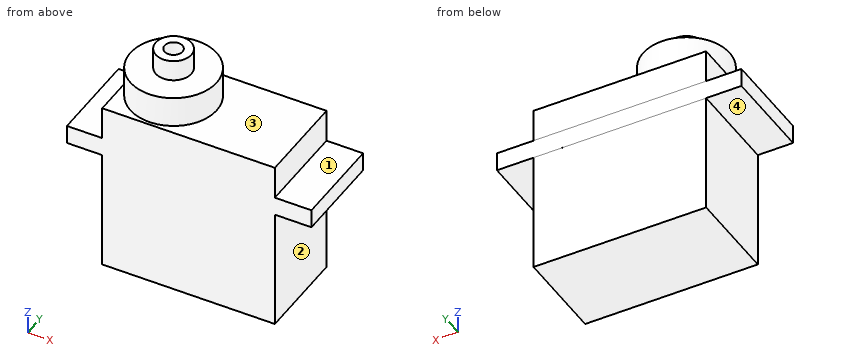
Solid Edge part; units mm, degrees
sketch "Sketch1" plane through (0, 0, 0) normal (0, 0, 1) x (1, 0, 0)
  line L0 (3.8592, 44.8625) -> (26.6354, 44.8625)
  line L1 (26.6354, 44.8625) -> (26.6354, 57.0462)
  line L2 (3.8592, 57.0462) -> (26.6354, 57.0462)
  line L3 (3.8592, 44.8625) -> (3.8592, 57.0462)
extrude "Ajout_matière_1" add sketch "Sketch1" against normal blind 16.002 and the other way blind 6.858
sketch "Sketch2" plane through (26.6354, 50.9544, -4.572) normal (1, 0, 0) x (0, 1, 0)
  line L0 (-5.4864, 7.0592) -> (6.0919, 7.0592)
  line L1 (6.0919, 7.0592) -> (6.0919, 4.572)
  line L2 (6.0919, 4.572) -> (-6.0919, 4.572)
  line L3 (-6.0919, 4.572) -> (-6.0919, 7.0592)
  line L4 (-6.0919, 7.0592) -> (-5.4864, 7.0592)
extrude "Ajout_matière_2" add sketch "Sketch2" along normal blind 4.826 and the other way blind 27.432
sketch "Sketch3" plane through (15.2473, 50.9544, 6.858) normal (0, 0, 1) x (1, 0, 0)
  circle A0 centre (-5.3803, 0) radius 5.6949
extrude "Ajout_matière_3" add sketch "Sketch3" along normal blind 4.064
sketch "Sketch4" plane through (9.867, 50.9544, 10.922) normal (0, 0, 1) x (1, 0, 0)
  circle A0 centre (0, 0) radius 2.3522
  circle A1 centre (0, 0) radius 1.1834
extrude "Ajout_matière_4" add sketch "Sketch4" along normal blind 2.794
properties part number "AC_1.14"
For this review, take the finished solid that the model builds, in its own axes (mm). Face numbers are marked on the shaded views. A direction names the side the tool comes from. Round coordinates to 2 decimals unless told otherwise and drop trailing zeros. Loops run counter-clockwise (first coordinate to the right, second up) from the corner with the lowest first, then second, coordinate; pieces in that order, holes last. Notation, with made-up numbers: (25, 27.5) - (71, 27.5) arc R31 ccw to (71, 60.5) - close; hole circle Ø1 at (-14, 29). An arc over 180 degrees is marked (long way). Use one line per item in the form item = value.
1) We need section B-B on y = 55. Write out the cut boundary in (x, z), then the cut area to 3 significant figures.
Solutions:
outline = (-0.8, 0) - (3.86, 0) - (3.86, -16) - (26.64, -16) - (26.64, 0) - (31.46, 0) - (31.46, 2.49) - (26.64, 2.49) - (26.64, 6.86) - (13.88, 6.86) - (13.88, 10.92) - (5.86, 10.92) - (5.86, 6.86) - (3.86, 6.86) - (3.86, 2.49) - (-0.8, 2.49) - close
area = 577 mm2
2) We need section C-C on z = -12. Write out the cut boundary in (x, y), then the cut area to 3 significant figures.
Solutions:
outline = (3.86, 44.86) - (26.64, 44.86) - (26.64, 57.05) - (3.86, 57.05) - close
area = 277 mm2
3) Wall thickness on probe 1 along Z at (x, y) = (27.5, 47.75); probe 2 along X at (y, z) = (54.5, 6.5); probe 3 along Z at (x, y) = (8, 53): over which ranges is each line inside the solid? List them lowest first.
Solutions:
probe_1 = 0 to 2.49
probe_2 = 3.86 to 26.64
probe_3 = -16 to 10.92
4) Tool access review of the marked faces 1, 2, 3 and 4: name each direction out of +Z, -Z, +X, -X, +Y, -Y from which nothing blocks a thin tool from reaching the whole face with its end or side.
Solutions:
face_1 = +Z, +Y, -Y
face_2 = -Z, +X, +Y, -Y
face_3 = +Z
face_4 = -Z, +Y, -Y
5) Clearance check with flat-ended pins moving along their axes: P1, Ø1, axis at y = 51.5, z = -4, coming from the +X side; P2, Ø1.2, axis at x = 9.5, y = 51, coming from the +Z side; P3, Ø1.5, axis at y = 48, z = -3, coming from the -X side. State where each tip first meets the part, or that it passes through.
Solutions:
P1 = 26.64
P2 = 10.92
P3 = 3.86
